Source: CAD feature listing. Evaluate the final solid. Frame: model axes, mm. Face numbers are marked on the shaded views. A direction names the side the tool comes from. Give positions to 0.01 mm unless a question says otherwise; leave off trailing zeros. Write each loop counter-clockwise with the first axis right and the second up, starting at its lowest first coordinate (ties: lowest second). Pieces come first, ordered by that corner, then holes.
```python
from build123d import *

# Parameters (mm, degrees)
FILLET_1_R          = 0.5
FILLET_2_R          = 1
CUT_EXTRUDE_1_DEPTH = 2.5
CHAMFER_1_SIZE      = 0.5
CHAMFER_1_SIZE2     = 0.866025404


with BuildPart() as part:
    # 草图1 → 旋转1 (revolve)
    with BuildSketch(Plane.XY):
        Polygon((7.5, 0), (-7.5, 0), (-7.5, 6), (-5.6, 6), (-2.6, 3), (7.5, 3), align=None)
    revolve(axis=Axis((7.5, 0, 0), (-1, 0, 0)))

    # 圆角1
    fillet_1_edges = [part.edges().sort_by_distance(p)[0] for p in [
        (-7.5, -6, 0),
    ]]
    fillet(fillet_1_edges, radius=FILLET_1_R)

    # 圆角2
    fillet_2_edges = [part.edges().sort_by_distance(p)[0] for p in [
        (-5.6, -6, 0),
    ]]
    fillet(fillet_2_edges, radius=FILLET_2_R)

    # 草图2 → 切除-拉伸1 (cut)
    with BuildSketch(Plane.ZY.offset(7.5)):
        Polygon((0, 2.309401077), (-2, 1.154700538), (-2, -1.154700538), (0, -2.309401077), (2, -1.154700538), (2, 1.154700538), align=None)
    extrude(amount=-CUT_EXTRUDE_1_DEPTH, mode=Mode.SUBTRACT)

    # 倒角1
    chamfer_1_edges = [part.edges().sort_by_distance(p)[0] for p in [
        (7.5, -3, 0),
    ]]
    chamfer_1_side = [part.faces().sort_by_distance(p)[0] for p in [
        (2.45, -3, 0),
    ]]
    chamfer(chamfer_1_edges, length=CHAMFER_1_SIZE, length2=CHAMFER_1_SIZE2, reference=chamfer_1_side[0])


solid = part.part
```
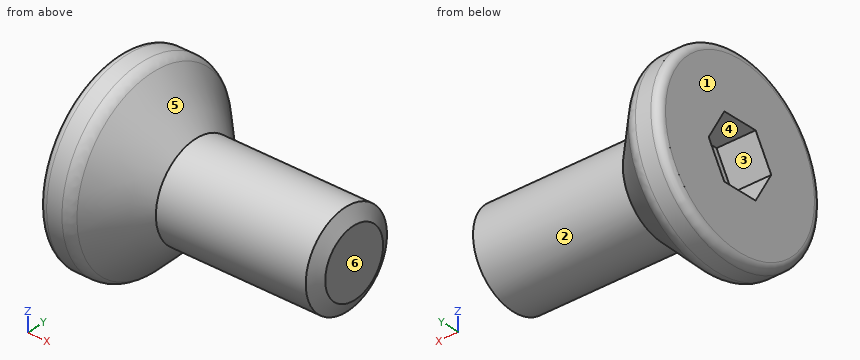
1. Cut plane A-A, the plane x = 4.75. Return the cut outline in (y, z), then the cut area to 3 significant figures.
2. Contact query for flat-ended pins moving along their axis: P1, Ø2, axis at x = -5, y = -3.5, coming from the +Z side; P2, Ø3, axis at x = -3, z = -1, coming from the +Y side; P3, Ø2, axis at y = 0.5, z = 0, coming from the -X side. Output: stop coordinate, or through.
3. Access query for the marked faces 1, 2 and 3. Directions: +Z, -Z, +X, -X, +Y, -Y. A direction counts if a zero-diameter tool reaches every point of the face in a straight line with its end or side. Return the directions, or none.
4. Line query: L1, parallel to X at y = -4.25, z = 1.75; L2, parallel to Y at x = 0, z = 1.75; L3, parallel to Y at x = 1, z = 1. Output: solid intervals per line, ascending.
5. Mould query, pull axis Z, two halves, no side actions, for the marked faces 4, 5 and 6. Classes: +Z half, -Z half, draft (parallel to the pull), parting line (faces both ways), or undercut.
Response values:
1. outline: circle Ø6 at (0, 0)
1. area: 28.3 mm2
2. P1: stops at z = 5.26
2. P2: stops at y = 4.82
2. P3: stops at x = -5
3. face 1: +Z, -Z, -X, +Y, -Y
3. face 2: +X
3. face 3: -X
4. L1: x = -7.5 to -4.2
4. L2: y = -2.44 to 2.44
4. L3: y = -2.83 to 2.83
5. face 4: undercut
5. face 5: parting line
5. face 6: draft
